Geometry: final body of the model. Coordinates: model frame, mm. Coordinates: 2 decimals unless noted, no trailing zeros. Write each loop counter-clockwise with the first axis right and the second up, starting at its lowest first coordinate (ties: lowest second). Pieces come first, ordered by that corner, then holes. Notation, with made-up numbers: (44.5, 83.25) -> (74.5, 83.25) arc R28 cw to (74.5, 112.25) -> close; hole circle Ø1 at (-1.5, 53). An arc over 180 degrees is marked (long way). One line per item, written item: value.
Autodesk Inventor part; units mm, degrees
ref_plane "YZ Plane" through (0, 0, 0) normal (1, 0, 0) x (0, 1, 0)
ref_plane "XZ Plane" through (0, 0, 0) normal (0, 1, 0) x (-1, 0, 0)
ref_plane "XY Plane" through (0, 0, 0) normal (0, 0, 1) x (1, 0, 0)
sketch "Sketch1" plane through (0, 0, 0) normal (1, 0, 0) x (0, 1, 0)
  line L0 (0, 0) -> (152.4, 0)
  line L1 (152.4, 0) -> (152.4, -295.275)
  line L2 (152.4, -295.275) -> (0, -295.275)
  line L3 (0, -295.275) -> (0, 0)
  line L4 (152.4, -295.275) -> (139.7, 0)
  line L5 (0, -9.525) -> (9.525, -9.525)
  line L6 (9.525, -9.525) -> (9.525, -19.05)
  line L7 (9.525, -19.05) -> (0, -19.05)
  line L8 (0, -19.05) -> (0, -9.525)
  point P0 (0, -19.05)
  dimension "d0" = 152.4
  dimension "d1" = 295.275
  dimension "d2" = 12.7
  dimension "d3" = 9.525
  dimension "d4" = 9.525
  dimension "d5" = 9.525
extrude "Extrusion1" add sketch "Sketch1" along normal blind 447.675 contours L0 L4 L2 L3 L7 L6 L5
equation "\"d5\" = d3"
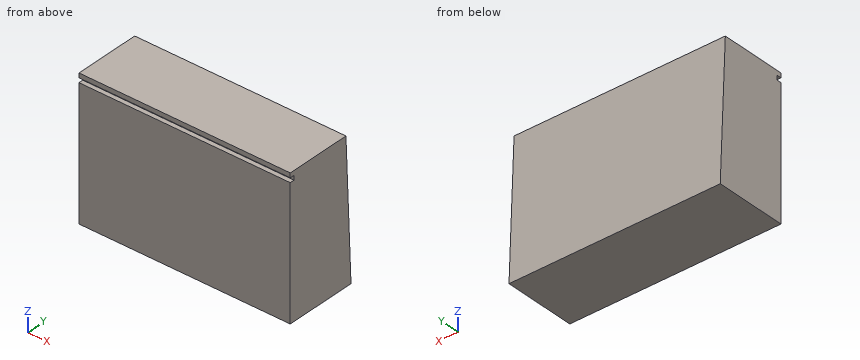
(1) Section B-B (z = -164). Return the cut outline in (x, y) (3 decimals), then the cut area to 3 significant figures.
Responses:
outline: (0, 0) -> (447.675, 0) -> (447.675, 146.754) -> (0, 146.754) -> close
area: 65,700 mm2
(2) Section A-A (x = 241). Return the cut outline in (y, z) (3 decimals).
Responses:
outline: (0, -295.275) -> (152.4, -295.275) -> (139.7, 0) -> (0, 0) -> (0, -9.525) -> (9.525, -9.525) -> (9.525, -19.05) -> (0, -19.05) -> close
(3) Line query: line 1 (Y direction, x = 222.5, z = -195.5); line 2 (Y direction, x = 393.5, z = -42.5). Output: solid intervals per line, ascending. Write a range as [from, to].
Responses:
line 1: y = [0, 148.11]
line 2: y = [0, 141.53]
(4) Section C-C (z = -35). Return the cut outline in (x, y) (3 decimals).
Responses:
outline: (0, 0) -> (447.675, 0) -> (447.675, 141.205) -> (0, 141.205) -> close
(5) First-contact query: pin 1 (6 mm diameter, centred on x = 281.5, z = -244.5, fed in from +Y); pin 2 (8 mm diameter, centred on x = 96.5, z = -137, fed in from +Y); pin 3 (3 mm diameter, centred on x = 219.5, z = -33.5, fed in from +Y). Flat tips, straight axial feed; report the tip coordinate or a pass-through.
Responses:
pin 1: stops at y = 150.35
pin 2: stops at y = 145.76
pin 3: stops at y = 141.21
